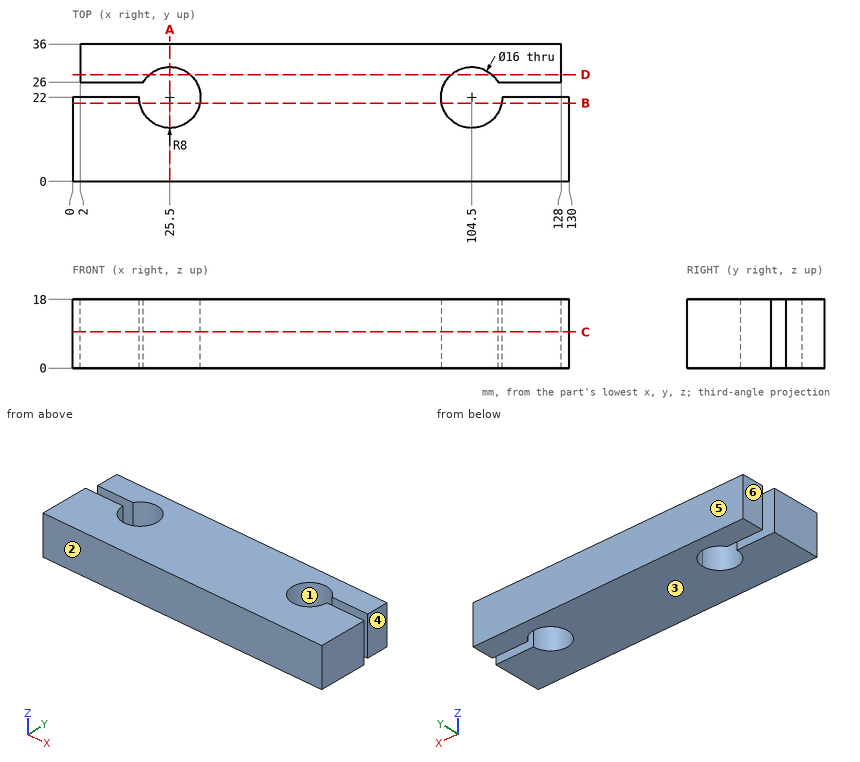
Can you work these out from the drawing? Everything is in mm from the part's minimum corner. A direction names the side the tool comes from. Coordinates: 2 decimals unless noted, no trailing zeros. Loops run counter-clockwise (first coordinate to the right, second up) from the corner with the lowest first, then second, coordinate; pieces in that order, holes last.
1. Imagine slicing it at C-C, the plane z = 9.5. Please give me the cut outline in (x, y).
2. Imagine slicing it at D-D, the plane y = 28. Please give me the cut outline in (x, z), and give its area (3 significant figures).
3. Imagine slicing it at B-B, the plane y = 20.5. Please give me the cut outline in (x, z), and give its area (3 significant figures).
4. Imagine slicing it at A-A, the plane x = 25.5. Please give me the cut outline in (y, z).
5. For P1, Ø13, axis at x = 104.5, y = 22, coming from the -Z side, with a flat end and sliding along its axis, tell me the tip position at first contact or that it passes through.
6. For the marked faces 4, 5 and 6, which set-ups out of +Z, -Z, +X, -X, +Y, -Y let a thin tool reach every point of the face, with its end or its side?
7. I need wall thicknesses on L1, parallel to Y at x = 104.5, z = 6.5; L2, parallel to Y at x = 116.5, z = 2.25; L3, parallel to X at y = 20, z = 3. Which ranges of each line are inside material? Lowest first, please.
8. If we mould it in two halves opening along Y, with no side actions, what happens to the marked faces 1, 2 and 3? For each: pulls with the +Y half, pulls with the -Y half, needs draft (parallel to the pull), parting line crosses it, or undercut.
Taken from the geometry:
1. outline: (0, 0) - (130, 0) - (130, 22) - (112.5, 22) arc R8 cw (long way) to (111.43, 26) - (128, 26) - (128, 36) - (2, 36) - (2, 26) - (18.57, 26) arc R8 cw (long way) to (17.5, 22) - (0, 22) - close
2. outline: (2, 0) - (20.21, 0) - (20.21, 18) - (2, 18) - close; (30.79, 0) - (99.21, 0) - (99.21, 18) - (30.79, 18) - close; (109.79, 0) - (128, 0) - (128, 18) - (109.79, 18) - close
2. area: 1,890 mm2
3. outline: (0, 0) - (17.64, 0) - (17.64, 18) - (0, 18) - close; (33.36, 0) - (96.64, 0) - (96.64, 18) - (33.36, 18) - close; (112.36, 0) - (130, 0) - (130, 18) - (112.36, 18) - close
3. area: 1,770 mm2
4. outline: (0, 0) - (14, 0) - (14, 18) - (0, 18) - close; (30, 0) - (36, 0) - (36, 18) - (30, 18) - close
5. P1: passes through
6. face 4: +Z, -Z, +X, +Y
6. face 5: +Z, -Z, +X, -X, +Y
6. face 6: +Z, -Z, -X, +Y
7. L1: y = 0 to 14, 30 to 36
7. L2: y = 0 to 22, 26 to 36
7. L3: x = 0 to 17.75, 33.25 to 96.75, 112.25 to 130
8. face 1: undercut
8. face 2: pulls with the -Y half
8. face 3: needs draft
